Can you work these out from the model? Positions are in its coordinate system, mm. A direction names the side the tool comes from. Give positions to 0.01 mm unless a question says otherwise; leave off trailing zeros. Write each loop counter-clockwise with the first axis right and the second up, starting at its lowest first coordinate (ties: lowest second). Pieces come first, ordered by that corner, then holes. Notation, with made-up numbers: M -9.75,-17 L 35.25,-17 A36 cw 35.25,18 Z; hole C 60,57 d3. An arc over 180 degrees is marked long. Write each question's results on one line, items separated by ' | '.
from build123d import *

# Parameters (mm, degrees)
SKETCH2_W            = 84
SKETCH2_H            = 24
BOSS_EXTRUDE1_DEPTH  = 1.5
SKETCH3_W            = 84
SKETCH3_H            = 24
SKETCH3_W_2          = 81
SKETCH3_H_2          = 21
BOSS_EXTRUDE2_DEPTH  = 2
CUT_EXTRUDE1_REACH   = 45.821
SKETCH4_R            = 1
SKETCH5_W            = 72.6
SKETCH5_H            = 17
CUT_EXTRUDE2_DEPTH   = 44.726422218
SKETCH8_W            = 24
SKETCH8_H            = 1.25
BOSS_EXTRUDE4_DEPTH  = 2
FILLET1_R            = 0.5
FILLET1_OF_MIRROR1_R = 0.5
SKETCH9_W            = 24
SKETCH9_H            = 41.5
BOSS_EXTRUDE5_DEPTH  = 1.5
BOSS_EXTRUDE6_DEPTH  = 2
SKETCH11_R           = 1
CUT_EXTRUDE4_DEPTH   = 70.298268377
SKETCH12_W           = 17
SKETCH12_H           = 36
CUT_EXTRUDE5_DEPTH   = 70.298268377
SKETCH13_W           = 11
SKETCH13_H           = 5.5
CUT_EXTRUDE6_DEPTH   = 1.5


with BuildPart() as part:
    # Sketch2 → Boss-Extrude1 (new body)
    with BuildSketch(Plane(origin=(0, 0, 0), x_dir=(1, 0, 0), z_dir=(0, 1, 0))):
        Rectangle(SKETCH2_W, SKETCH2_H)
    extrude(amount=BOSS_EXTRUDE1_DEPTH)

    # Sketch3 → Boss-Extrude2 (add)
    with BuildSketch(Plane(origin=(0, 1.5, 0), x_dir=(1, 0, 0), z_dir=(0, 1, 0))):
        Rectangle(SKETCH3_W, SKETCH3_H)
        Rectangle(SKETCH3_W_2, SKETCH3_H_2, mode=Mode.SUBTRACT)
    extrude(amount=BOSS_EXTRUDE2_DEPTH)

    # Sketch4 → Cut-Extrude1 (cut, up to next)
    with BuildSketch(Plane.XZ, mode=Mode.PRIVATE) as cut_extrude1_sk1:
        with Locations(Location((-37.955, 8.005, 0), (0, 0, 270))):
            Circle(SKETCH4_R)
    cut_extrude1_tool1 = extrude(cut_extrude1_sk1.sketch, amount=-CUT_EXTRUDE1_REACH, mode=Mode.PRIVATE) & part.part
    # Sketch4 → Cut-Extrude1 (cut, up to next)
    with BuildSketch(Plane.XZ, mode=Mode.PRIVATE) as cut_extrude1_sk2:
        with Locations(Location((37.955, 8.005, 0), (0, 0, 270))):
            Circle(SKETCH4_R)
    cut_extrude1_tool2 = extrude(cut_extrude1_sk2.sketch, amount=-CUT_EXTRUDE1_REACH, mode=Mode.PRIVATE) & part.part
    # Sketch4 → Cut-Extrude1 (cut, up to next)
    with BuildSketch(Plane.XZ, mode=Mode.PRIVATE) as cut_extrude1_sk3:
        with Locations(Location((37.955, -8.005, 0), (0, 0, 270))):
            Circle(SKETCH4_R)
    cut_extrude1_tool3 = extrude(cut_extrude1_sk3.sketch, amount=-CUT_EXTRUDE1_REACH, mode=Mode.PRIVATE) & part.part
    # Sketch4 → Cut-Extrude1 (cut, up to next)
    with BuildSketch(Plane.XZ, mode=Mode.PRIVATE) as cut_extrude1_sk4:
        with Locations(Location((-37.955, -8.005, 0), (0, 0, 270))):
            Circle(SKETCH4_R)
    cut_extrude1_tool4 = extrude(cut_extrude1_sk4.sketch, amount=-CUT_EXTRUDE1_REACH, mode=Mode.PRIVATE) & part.part
    add(cut_extrude1_tool1.solids().sort_by_distance((-37.955, 0, 8.005))[0], mode=Mode.SUBTRACT)
    add(cut_extrude1_tool2.solids().sort_by_distance((37.955, 0, 8.005))[0], mode=Mode.SUBTRACT)
    add(cut_extrude1_tool3.solids().sort_by_distance((37.955, 0, -8.005))[0], mode=Mode.SUBTRACT)
    add(cut_extrude1_tool4.solids().sort_by_distance((-37.955, 0, -8.005))[0], mode=Mode.SUBTRACT)

    # Sketch5 → Cut-Extrude2 (cut, through all)
    with BuildSketch(Plane(origin=(0, 1.5, 0), x_dir=(1, 0, 0), z_dir=(0, 1, 0))):
        Rectangle(SKETCH5_W, SKETCH5_H)
    extrude(amount=-CUT_EXTRUDE2_DEPTH, mode=Mode.SUBTRACT)

    # Sketch8 → Boss-Extrude4 (add)
    with BuildSketch(Plane(origin=(42, 0, 0), x_dir=(0, 0, -1), z_dir=(1, 0, 0))):
        with Locations((0, 1.75)):
            Rectangle(SKETCH8_W, SKETCH8_H)
    boss_extrude4 = extrude(amount=BOSS_EXTRUDE4_DEPTH)

    # Fillet1
    fillet1_edges = [part.edges().sort_by_distance(p)[0] for p in [
        (43, 1.125, -12),
        (43, 2.375, -12),
        (43, 2.375, 12),
        (43, 1.125, 12),
        (44, 1.75, -12),
        (44, 2.375, 0),
        (44, 1.75, 12),
        (44, 1.125, 0),
    ]]
    fillet(fillet1_edges, radius=FILLET1_R)

    # Mirror1: Boss-Extrude4 across plane
    add(boss_extrude4.mirror(Plane(origin=(0, 0, 0), x_dir=(0, 0, 1), z_dir=(1, 0, 0))))

    # Fillet1 of Mirror1
    fillet1_of_mirror1_edges = [part.edges().sort_by_distance(p)[0] for p in [
        (-43, 1.125, -12),
        (-43, 2.375, -12),
        (-43, 2.375, 12),
        (-43, 1.125, 12),
        (-44, 1.75, -12),
        (-44, 2.375, 0),
        (-44, 1.75, 12),
        (-44, 1.125, 0),
    ]]
    fillet(fillet1_of_mirror1_edges, radius=FILLET1_OF_MIRROR1_R)

    # Sketch9 → Boss-Extrude5 (add)
    with BuildSketch(Plane(origin=(0, 0, 0), x_dir=(1, 0, 0), z_dir=(0, 1, 0))):
        with Locations((-6, -32.75)):
            Rectangle(SKETCH9_W, SKETCH9_H)
    extrude(amount=BOSS_EXTRUDE5_DEPTH)

    # Sketch10 → Boss-Extrude6 (add)
    with BuildSketch(Plane(origin=(0, 1.5, 0), x_dir=(1, 0, 0), z_dir=(0, 1, 0))):
        Polygon((-16.5, -52), (-16.5, -13.5), (-16.5, -12), (-18, -12), (-18, -53.5), (6, -53.5), (6, -12), (4.5, -12), (4.5, -13.5), (4.5, -52), align=None)
    extrude(amount=BOSS_EXTRUDE6_DEPTH)

    # Sketch11 → Cut-Extrude4 (cut, through all)
    with BuildSketch(Plane(origin=(0, 1.5, 0), x_dir=(1, 0, 0), z_dir=(0, 1, 0))):
        with Locations(Location((-14, -49.45, 0), (0, 0, 270))):
            Circle(SKETCH11_R)
        with Locations(Location((2, -49.45, 0), (0, 0, 270))):
            Circle(SKETCH11_R)
    extrude(amount=-CUT_EXTRUDE4_DEPTH, mode=Mode.SUBTRACT)

    # Sketch12 → Cut-Extrude5 (cut, through all)
    with BuildSketch(Plane(origin=(0, 1.5, 0), x_dir=(1, 0, 0), z_dir=(0, 1, 0))):
        with Locations((-6, -30)):
            Rectangle(SKETCH12_W, SKETCH12_H)
    extrude(amount=-CUT_EXTRUDE5_DEPTH, mode=Mode.SUBTRACT)

    # Sketch13 → Cut-Extrude6 (cut)
    with BuildSketch(Plane.XZ):
        with Locations((-6, 50.75)):
            Rectangle(SKETCH13_W, SKETCH13_H)
    extrude(amount=-CUT_EXTRUDE6_DEPTH, mode=Mode.SUBTRACT)


solid = part.part
Item 1: I want a section at D-D, the plane x = 16.5. Please give me the cut outline in (y, z), and give its area (3 significant figures).
Geometry says:
outline: M 0,-12 L 3.5,-12 L 3.5,-10.5 L 1.5,-10.5 L 1.5,-8.5 L 0,-8.5 Z; M 0,8.5 L 1.5,8.5 L 1.5,10.5 L 3.5,10.5 L 3.5,12 L 0,12 Z | area: 16.5 mm2
Item 2: Thinking about a two-plate mould opening in X: for faces 1 (the face through (40.5, 2, 0)), 2 (the face through (-18, 2, 32)), 3 (the face through (-40.5, 2, 0)), 4 (the face through (24, 2, 12)), which applies, +X half, -X half, draft (parallel to the pull), parting line (faces both ways), or undercut?
Geometry says:
face 1: undercut | face 2: -X half | face 3: undercut | face 4: draft
Item 3: For faces 5 (the face through (-16.5, 2, 32)), 6 (the face through (-6, 3.5, 11)), 7 (the face through (-31, 2, 12)), which set-ups out of +Z, -Z, +X, -X, +Y, -Y let a thin tool reach every point of the face, with its end or its side?
Geometry says:
face 5: +Y | face 6: +Z, -Z, +X, -X, +Y | face 7: +Z, -X, +Y, -Y
Item 4: I want a section at A-A, the plane x = -5.5. Please give me the cut outline in (y, z), and give its area (3 significant figures).
Geometry says:
outline: M 0,-12 L 3.5,-12 L 3.5,-10.5 L 1.5,-10.5 L 1.5,-8.5 L 0,-8.5 Z; M 0,8.5 L 1.5,8.5 L 1.5,10.5 L 3.5,10.5 L 3.5,12 L 0,12 Z; M 1.5,52 L 3.5,52 L 3.5,53.5 L 1.5,53.5 Z | area: 19.5 mm2
Item 5: I want a section at C-C, the plane z = 49.45. Please give me the cut outline in (x, y).
Geometry says:
outline: M -18,0 L -15,0 L -15,1.5 L -16.5,1.5 L -16.5,3.5 L -18,3.5 Z; M -13,0 L -11.5,0 L -11.5,1.5 L -13,1.5 Z; M -0.5,0 L 1,0 L 1,1.5 L -0.5,1.5 Z; M 3,0 L 6,0 L 6,3.5 L 4.5,3.5 L 4.5,1.5 L 3,1.5 Z
Item 6: I want a section at B-B, the plane z = 22. Please give me the cut outline in (x, y), and give its area (3 significant figures).
Geometry says:
outline: M -18,0 L -14.5,0 L -14.5,1.5 L -16.5,1.5 L -16.5,3.5 L -18,3.5 Z; M 2.5,0 L 6,0 L 6,3.5 L 4.5,3.5 L 4.5,1.5 L 2.5,1.5 Z | area: 16.5 mm2
Item 7: If I drill on line 1 (Z direction, x = -13.5, y = 2.35); line 2 (X direction, y = 0.85, z = 25); line 3 (X direction, y = 1.65, z = 14), over which ranges is the centre line in solid material (lowest first)? Write a range as from..to.
Geometry says:
line 1: z = -12..-10.5, 10.5..12, 52..53.5 | line 2: x = -18..-14.5, 2.5..6 | line 3: x = -18..-16.5, 4.5..6
Item 8: I'm going to push flat-ended pins straight in: pin 1 (1.6 mm diameter, centred on y = 3, z = -5, fed in from -X); pin 2 (0.8 mm diameter, centred on y = 1, z = 52, fed in from -X); pin 3 (0.6 mm diameter, centred on y = 2.5, z = -2, fed in from +X); pin 4 (1.3 mm diameter, centred on y = 2.5, z = 2, fed in from +X). Where does each tip first touch, or does it pass through?
Geometry says:
pin 1: stops at x = -43.88 | pin 2: stops at x = -18 | pin 3: stops at x = 43.88 | pin 4: stops at x = 44
